Could you check a few things on this drawing? It's one solid part, dimensions in mm from its lowest x, y, z. Round coordinates to 2 decimals unless told otherwise and drop trailing zeros. Loops run counter-clockwise (first coordinate to the right, second up) from the corner with the lowest first, then second, coordinate; pieces in that order, holes last. Notation, with made-up numbers: M 87.5,71 L 102.5,71 A23 cw 102.5,94 Z; hole C 35.25,81 d3. An arc over 180 degrees is marked long. Write item = value, one per line. Start each with the question number.
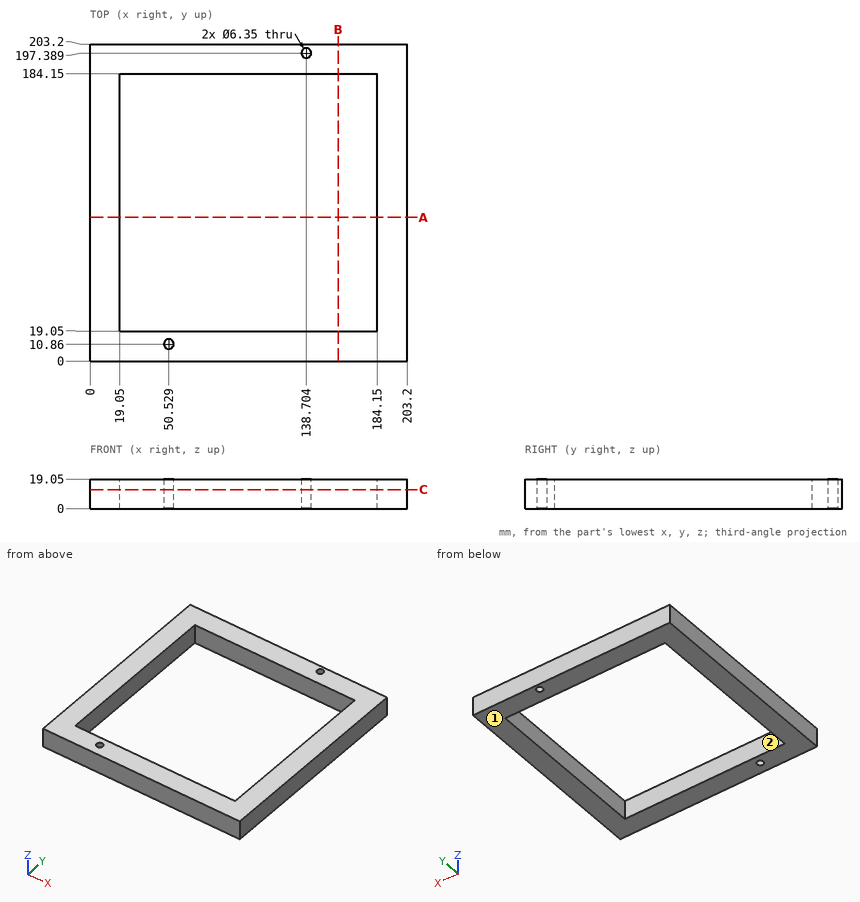
Item 1: I want a section at C-C, the plane z = 12.25. State how many separate pieces and enclosed holes the cut face has, then the cut area to 3 significant figures.
Item 2: Please list where these lines run through material, in increasing order: line 1 (Y direction, x = 32, z = 8.5); line 2 (X direction, y = 9.5, z = 18). Write a range as [from, to].
Item 3: We'd pull the mould along X, two halves only. Please class the marked faces 1 and 2: released by +X, released by -X, zero draft, split by the parting line, or undercut.
Item 4: I want a section at A-A, the plane y = 92. List the corners of the cut face in (x, z) for me, then the cut area to 3 significant figures.
Worked out:
q1.separate_pieces = 1
q1.enclosed_holes = 3
q1.area = 14,000 mm2
q2.line_1 = [0, 19.05], [184.15, 203.2]
q2.line_2 = [0, 47.66], [53.4, 203.2]
q3.face_1 = zero draft
q3.face_2 = undercut
q4.outline = M 0,0 L 19.05,0 L 19.05,19.05 L 0,19.05 Z; M 184.15,0 L 203.2,0 L 203.2,19.05 L 184.15,19.05 Z
q4.area = 726 mm2
